```python
from build123d import *

# Parameters (mm, degrees)
ESBO_O2_R                  = 2.5
CORTE_EXTRUS_O1_DEPTH      = 20
RESSALTO_EXTRUS_O1_DEPTH   = 8.5
CORTE_EXTRUS_O2_DEPTH      = 10
CORTE_EXTRUS_O2_DEPTH_BACK = 10
ESBO_O5_R                  = 1.5


with BuildPart() as part:
    # Esboço1 → Revolução1 (revolve)
    with BuildSketch(Plane.XY):
        Polygon((0, 17.5), (0, 0), (-5, 0), (-9, 0), (-9, 8), (-9, 9), (-5, 9), (-5, 16.5), (-9, 16.5), (-9, 17.5), align=None)
    revolve(axis=Axis((0, 17.5, 0), (0, -1, 0)))

    # Esboço2 → Corte-extrusão1 (cut)
    with BuildSketch(Plane(origin=(0, 17.5, 0), x_dir=(1, 0, 0), z_dir=(0, 1, 0))):
        with Locations(Location((0, 0, 0), (0, 0, 180))):
            Circle(ESBO_O2_R)
    extrude(amount=-CORTE_EXTRUS_O1_DEPTH, mode=Mode.SUBTRACT)

    # Esboço4 → Ressalto-extrusão1 (add)
    with BuildSketch(Plane(origin=(0, 17.5, 0), x_dir=(1, 0, 0), z_dir=(0, 1, 0))):
        Polygon((0.75, 2.711240108), (0.539299188, 2.711240108), (1.535794152, 2.298478379), (1.38680618, 2.447466352), (2.135819299, 3.196479471), (3.167059402, 5.686113314), (1.781240103, 6.260138462), (0.75, 3.770504619), align=None)
        Polygon((1.73045632, 2.217846669), (1.535794152, 2.298478379), (2.298478379, 1.535794152), (2.217846669, 1.73045632), (3.196479471, 2.135819299), (5.101962719, 4.041302547), (4.041302547, 5.101962719), (2.135819299, 3.196479471), align=None)
        Polygon((2.447466352, 1.38680618), (2.298478379, 1.535794152), (2.711240108, 0.539299188), (2.711240108, 0.75), (3.770504619, 0.75), (6.260138462, 1.781240103), (5.686113314, 3.167059402), (3.196479471, 2.135819299), align=None)
        Polygon((0.539299188, 2.711240108), (0.344637021, 2.791871818), (0.75, 3.770504619), (0.75, 6.465264872), (-0.75, 6.465264872), (-0.75, 3.770504619), (-0.344637021, 2.791871818), (-0.539299188, 2.711240108), align=None)
        Polygon((-1.535794152, 2.298478379), (-0.539299188, 2.711240108), (-0.75, 2.711240108), (-0.75, 3.770504619), (-1.781240103, 6.260138462), (-3.167059402, 5.686113314), (-2.135819299, 3.196479471), (-1.38680618, 2.447466352), align=None)
        Polygon((-2.298478379, 1.535794152), (-1.535794152, 2.298478379), (-1.73045632, 2.217846669), (-2.135819299, 3.196479471), (-4.041302547, 5.101962719), (-5.101962719, 4.041302547), (-3.196479471, 2.135819299), (-2.217846669, 1.73045632), align=None)
        Polygon((-2.711240108, 0.539299188), (-2.298478379, 1.535794152), (-2.447466352, 1.38680618), (-3.196479471, 2.135819299), (-5.686113314, 3.167059402), (-6.260138462, 1.781240103), (-3.770504619, 0.75), (-2.711240108, 0.75), align=None)
        Polygon((-2.711240108, -0.539299188), (-2.711240108, 0.539299188), (-2.791871818, 0.344637021), (-3.770504619, 0.75), (-6.465264872, 0.75), (-6.465264872, -0.75), (-3.770504619, -0.75), (-2.791871818, -0.344637021), align=None)
        Polygon((-2.298478379, -1.535794152), (-2.711240108, -0.539299188), (-2.711240108, -0.75), (-3.770504619, -0.75), (-6.260138462, -1.781240103), (-5.686113314, -3.167059402), (-3.196479471, -2.135819299), (-2.447466352, -1.38680618), align=None)
        Polygon((-1.535794152, -2.298478379), (-2.298478379, -1.535794152), (-2.217846669, -1.73045632), (-3.196479471, -2.135819299), (-5.101962719, -4.041302547), (-4.041302547, -5.101962719), (-2.135819299, -3.196479471), (-1.73045632, -2.217846669), align=None)
        Polygon((-0.539299188, -2.711240108), (-1.535794152, -2.298478379), (-1.38680618, -2.447466352), (-2.135819299, -3.196479471), (-3.167059402, -5.686113314), (-1.781240103, -6.260138462), (-0.75, -3.770504619), (-0.75, -2.711240108), align=None)
        Polygon((0.344637021, -2.791871818), (0.539299188, -2.711240108), (-0.539299188, -2.711240108), (-0.344637021, -2.791871818), (-0.75, -3.770504619), (-0.75, -6.465264872), (0.75, -6.465264872), (0.75, -3.770504619), align=None)
        Polygon((1.38680618, -2.447466352), (1.535794152, -2.298478379), (0.539299188, -2.711240108), (0.75, -2.711240108), (0.75, -3.770504619), (1.781240103, -6.260138462), (3.167059402, -5.686113314), (2.135819299, -3.196479471), align=None)
        Polygon((2.217846669, -1.73045632), (2.298478379, -1.535794152), (1.535794152, -2.298478379), (1.73045632, -2.217846669), (2.135819299, -3.196479471), (4.041302547, -5.101962719), (5.101962719, -4.041302547), (3.196479471, -2.135819299), align=None)
        Polygon((2.711240108, -0.75), (2.711240108, -0.539299188), (2.298478379, -1.535794152), (2.447466352, -1.38680618), (3.196479471, -2.135819299), (5.686113314, -3.167059402), (6.260138462, -1.781240103), (3.770504619, -0.75), align=None)
        Polygon((2.791871818, 0.344637021), (2.711240108, 0.539299188), (2.711240108, -0.539299188), (2.791871818, -0.344637021), (3.770504619, -0.75), (6.465264872, -0.75), (6.465264872, 0.75), (3.770504619, 0.75), align=None)
    extrude(amount=-RESSALTO_EXTRUS_O1_DEPTH)

    # Esboço5 → Corte-extrusão2 (cut, two sides: drawn at the far end of the back side and taken through both)
    with BuildSketch(Plane.XY.offset(-CORTE_EXTRUS_O2_DEPTH_BACK)):
        with Locations(Location((0, 4.5, 0), (0, 0, 180))):
            Circle(ESBO_O5_R)
    extrude(amount=CORTE_EXTRUS_O2_DEPTH + CORTE_EXTRUS_O2_DEPTH_BACK, mode=Mode.SUBTRACT)


solid = part.part
```
Geometry check sheet. Reference: the model listing, model coordinates, mm. A direction names the side the tool comes from. Give positions to 0.01 mm unless a question says otherwise; leave off trailing zeros. Order: outer loops, then holes, each group sorted by start corner. A loop starts at its lowest first (then second) coordinate and runs counter-clockwise, first axis right, second up. Notation, with made-up numbers: (10.5, 72.25) - (15.5, 72.25) arc R29 ccw to (15.5, 106.25) - close; hole circle Ø6 at (89, 44). An arc over 180 degrees is marked (long way). Answer in a Markdown table with one row per item. Add a question column.
Q1. Cross-section at B-B, the plane z = 0. Enter the section's corners in (x, y).
Q2. Cross-section at A-A, the plane x = 0. Enter the section's corners in (y, z).
Q3. Gauge pin test, flat ends, axial feed: pin 1 (1.2 mm diameter, centred on y = 13.5, z = 0.5, fed in from +X); pin 2 (5 mm diameter, centred on x = -1, y = 12.5, fed in from -Z); pin 3 (5 mm diameter, centred on x = -5, y = 12.5, fed in from -Z). Record the tip position at first contact, or that the pin passes through.
Q4. Material ranges on probe 1 along Y at (x, z) = (0, -6.5); probe 2 along X at (y, z) = (12.25, -4.5); probe 3 along Y at (x, z) = (-0.5, -7.5), recorded low to high. Write a range as from..to.
Q5. Cross-section at D-D, the plane z = 7. Enter the section's corners in (x, y).
Q6. Mould release check, pull along Z, two halves, no side actions. Record for faces 5 (the flat face through (1.486, 12.802, 5.547)), 6 (the flat face through (-2.88, 12.8, -4.99)), 7 (the flat face through (-2, 17.5, 2)): pulls with the +Z half, pulls with the -Z half, needs draft (parallel to the pull), parting line crosses it, or undercut.
Q7. Cross-section at C-C, the plane y = 4.5. Enter the section's corners in (x, z).
Q8. Tool access check on faces 1 (the flat face through (-4.99, 12.8, 2.88)), 2 (the flat face through (-6.465, 13, 0)), 3 (the flat face through (-1.486, 12.802, -5.547)), 4 (the flat face through (6.465, 13, 0)). Record the directions out of +Z, -Z, +X, -X, +Y, -Y that give a thin tool (end or side, any length) a straight path to the whole face; none if there is none.
Check values:
| question | item | result |
|---|---|---|
| 1 | outline | (-9, 0) - (-2.5, 0) - (-2.5, 17.5) - (-9, 17.5) - (-9, 16.5) - (-6.47, 16.5) - (-6.47, 9) - (-9, 9) - close; (2.5, 0) - (9, 0) - (9, 9) - (6.47, 9) - (6.47, 16.5) - (9, 16.5) - (9, 17.5) - (2.5, 17.5) - close |
| 2 | outline | (0, -9) - (3, -9) - (3, -2.5) - (0, -2.5) - close; (0, 2.5) - (3, 2.5) - (3, 9) - (0, 9) - close; (6, -9) - (9, -9) - (9, -6.47) - (16.5, -6.47) - (16.5, -9) - (17.5, -9) - (17.5, -2.5) - (6, -2.5) - close; (6, 2.5) - (17.5, 2.5) - (17.5, 9) - (16.5, 9) - (16.5, 6.47) - (9, 6.47) - (9, 9) - (6, 9) - close |
| 3 | pin 1 | stops at x = 6.47 |
| 3 | pin 2 | stops at z = -6.47 |
| 3 | pin 3 | stops at z = -5.96 |
| 4 | probe 1 | y = 0..3, 6..9, 16.5..17.5 |
| 4 | probe 2 | x = -4.64..-3.44, -2.68..2.68, 3.44..4.64 |
| 4 | probe 3 | y = 0..3.09, 5.91..9, 16.5..17.5 |
| 5 | outline | (-5.66, 0) - (5.66, 0) - (5.66, 9) - (-5.66, 9) - close; (-5.66, 16.5) - (5.66, 16.5) - (5.66, 17.5) - (-5.66, 17.5) - close; hole circle Ø3 at (0, 4.5) |
| 6 | face 5 | pulls with the +Z half |
| 6 | face 6 | undercut |
| 6 | face 7 | needs draft |
| 7 | outline | (-1.5, -8.87) - (-1.5, -2) arc R2.5 cw to (-1.5, 2) - (-1.5, 8.87) arc R9 ccw to start; (1.5, -8.87) arc R9 ccw to (1.5, 8.87) - (1.5, 2) arc R2.5 cw to (1.5, -2) - close |
| 8 | face 1 | none |
| 8 | face 2 | +Z, -Z, -X |
| 8 | face 3 | -Z |
| 8 | face 4 | +Z, -Z, +X |
